from build123d import *

# Parameters (mm, degrees)
PAD_DEPTH    = 20
FILLET_R     = 77
CHAMFER_SIZE = 3
FILLET001_R  = 3
FILLET002_R  = 4
FILLET003_R  = 8
FILLET004_R  = 6
FILLET005_R  = 5
FILLET006_R  = 5
FILLET007_R  = 4
FILLET008_R  = 7
FILLET009_R  = 3


with BuildPart() as part:
    # Sketch → Pad (new body)
    with BuildSketch(Plane.XY):
        Polygon((0, 0), (59.950146, 0), (59.950146, -5), (11.518525, -5), (11.518525, -40.3), (60.519711, -40.3), (60.519711, -45.3), (15.353175, -45.3), (10.617641, -60.148293), (14.104488, -105.074165), (39.071716, -113.621506), (70.78685, -107.773331), (79.334183, -99.001053), (77.653412, -94.872163), (91.389916, -94.872163), (73.935867, -115.420944), (39.52158, -123.518425), (6.007014, -113.171646), (0.177902, -59.873554), (0.177902, -43.792206), align=None)
    extrude(amount=PAD_DEPTH)

    # Fillet
    fillet_edges = [part.edges().sort_by_distance(p)[0] for p in [
        (39.071716, -113.621506, 10),
        (39.52158, -123.518425, 10),
    ]]
    fillet(fillet_edges, radius=FILLET_R)

    # Chamfer
    chamfer_edges = [part.edges().sort_by_distance(p)[0] for p in [
        (14.104488, -105.074165, 10),
    ]]
    chamfer(chamfer_edges, length=CHAMFER_SIZE)

    # Fillet001
    fillet001_edges = [part.edges().sort_by_distance(p)[0] for p in [
        (79.334183, -99.001053, 10),
    ]]
    fillet(fillet001_edges, radius=FILLET001_R)

    # Fillet002
    fillet002_edges = [part.edges().sort_by_distance(p)[0] for p in [
        (70.78685, -107.773331, 10),
    ]]
    fillet(fillet002_edges, radius=FILLET002_R)

    # Fillet003
    fillet003_edges = [part.edges().sort_by_distance(p)[0] for p in [
        (73.935867, -115.420944, 10),
    ]]
    fillet(fillet003_edges, radius=FILLET003_R)

    # Fillet004
    fillet004_edges = [part.edges().sort_by_distance(p)[0] for p in [
        (91.389916, -94.872163, 10),
    ]]
    fillet(fillet004_edges, radius=FILLET004_R)

    # Fillet005
    fillet005_edges = [part.edges().sort_by_distance(p)[0] for p in [
        (6.007014, -113.171646, 10),
    ]]
    fillet(fillet005_edges, radius=FILLET005_R)

    # Fillet006
    fillet006_edges = [part.edges().sort_by_distance(p)[0] for p in [
        (13.872346, -102.08316, 10),
        (16.942774, -106.045831, 10),
    ]]
    fillet(fillet006_edges, radius=FILLET006_R)

    # Fillet007
    fillet007_edges = [part.edges().sort_by_distance(p)[0] for p in [
        (15.353175, -45.3, 10),
    ]]
    fillet(fillet007_edges, radius=FILLET007_R)

    # Fillet008
    fillet008_edges = [part.edges().sort_by_distance(p)[0] for p in [
        (10.617641, -60.148293, 10),
    ]]
    fillet(fillet008_edges, radius=FILLET008_R)

    # Fillet009
    fillet009_edges = [part.edges().sort_by_distance(p)[0] for p in [
        (0, 0, 10),
    ]]
    fillet(fillet009_edges, radius=FILLET009_R)


solid = part.part
Verification items for the finished model (mm, model axes). A direction names the side the tool comes from. Coordinates: 2 decimals unless noted, no trailing zeros. Order: outer loops, then holes, each group sorted by start corner. A loop starts at its lowest first (then second) coordinate and runs counter-clockwise, first axis right, second up. Notation, with made-up numbers: M 87,68.25 L 136,68.25 A33 cw 136,107.25 Z; hole C 40.5,-16.75 d4. An arc over 180 degrees is marked long. One line per item, written item: value. Start each with the question number.
Item 1: Sectioned sample at D-D (x = 74). Enter the section's corners in (y, z).
Item 2: Scan lines: probe 1 along Y at (x, z) = (27, 8.5); probe 2 along Y at (x, z) = (45, 9.5); probe 3 along X at (y, z) = (-8.5, 7.5). Record each from-to range of solid material in increasing order.
Item 3: Mould release check, pull along X, two halves, no side actions. Record for faces 1 (the cylindrical face through (17.09, -105.88, 10.14)), 2 (the flat face through (79.368, -109.025, 9.86)), 3 (the flat face through (31, 0, 10)), 4 (the flat face through (0.178, -52, 10)): released by +X, released by -X, zero draft, split by the parting line, or undercut.
Item 4: Gauge pin test, flat ends, axial feed: pin 1 (10 mm diameter, centred on y = -23.5, z = 7.5, fed in from -X); pin 2 (5.5 mm diameter, centred on y = -1.5, z = 10, fed in from +X); pin 3 (1.5 mm diameter, centred on y = -86, z = 11, fed in from -X); pin 4 (6 mm diameter, centred on x = 16.5, y = -78, fed in from -Z). Record the tip position at first contact, or that the pin passes through.
Item 5: Sectioned sample at C-C (y = -37). Enter the section's corners in (x, z).
Item 6: Sectioned sample at A-A (x = 42.5). Enter the section's corners in (y, z).
Item 7: Access from +Z, -Z, +X, -X, +Y, -Y to the whole of each face (thin tool, end or side, straight path). Record for faces 5 (the flat face through (2.952, -85.24, 9.86)), 6 (the cylindrical face through (38.988, -111.012, 10.14)), 7 (the flat face through (36, -40.3, 10)).
Conclusion:
1. outline: M -114.88,0 L -104.48,0 L -104.48,20 L -114.88,20 Z
2. probe 1: y = -119.25 to -109.12, -45.3 to -40.3, -5 to 0
2. probe 2: y = -120.72 to -111.24, -45.3 to -40.3, -5 to 0
2. probe 3: x = 0.03 to 11.52
3. face 1: undercut
3. face 2: released by +X
3. face 3: zero draft
3. face 4: released by -X
4. pin 1: stops at x = 0.08
4. pin 2: stops at x = 59.95
4. pin 3: stops at x = 2.95
4. pin 4: passes through
5. outline: M 0.15,0 L 11.52,0 L 11.52,20 L 0.15,20 Z
6. outline: M -120.77,0 L -111.2,0 L -111.2,20 L -120.77,20 Z; M -45.3,0 L -40.3,0 L -40.3,20 L -45.3,20 Z; M -5,0 L 0,0 L 0,20 L -5,20 Z
7. face 5: +Z, -Z, -X, -Y
7. face 6: +Z, -Z
7. face 7: +Z, -Z, +X
